The listing builds one solid part. Answer for the finished solid, in the listing's coordinates (mm). Face numbers are marked on the shaded views. A direction names the side the tool comes from. Give positions to 0.01 mm unless a question says otherwise; leave off trailing zeros. Order: outer loops, then holes, each group sorted by start corner. A loop starts at its lowest first (then second) coordinate and runs counter-clockwise, first axis right, second up. Notation, with made-up numbers: (-6.5, 53) - (-2.5, 53) arc R29 cw to (-2.5, 86) - close; hole circle Ø5 at (25, 85.25). An arc over 180 degrees is marked (long way). Use a Markdown table: item, result. Add a question column.
1) The mould has two halves that part along X. Classify the marked faces 5, 6 and 7: released by +X, released by -X, zero draft, split by the parting line, or undercut.
2) Find section D-D, the plane x = 17.5. Determine the outline of the cut face in (y, z), plus the area to 3 significant figures.
3) For the marked faces 1, 2, 3 and 4, determine the directions among +Z, -Z, +X, -X, +Y, -Y from which every point of the face is accessible in a straight line to the end or side of a thin tool.
4) Find section A-A, the plane x = 26.5. Determine the outline of the cut face in (y, z).
5) Find section C-C, the plane z = -4. Determine the outline of the cut face in (x, y).
6) Find section B-B, the plane z = -26.5. Determine the outline of the cut face in (x, y), plus the area to 3 significant figures.
7) Flat-ended cylindrical pins translate along their axes: pin 1 (10 mm diameter, centred on y = 18, z = -20.5, fed in from +X); pin 2 (16.5 mm diameter, centred on y = 11, z = -16.5, fed in from +X); pin 3 (1.5 mm diameter, centred on x = 46, y = 22, fed in from -Z); pin 4 (1.5 mm diameter, centred on x = 6, y = 18.5, fed in from -Z). Find the tip coordinate at first contact, or state that the pin passes through.
8) Straight lines are drawn through the part: line 1 (Z direction, x = 4, y = 4); line 2 (Z direction, x = 67, y = 6); line 3 (Z direction, x = 43.5, y = 19). For each, find the intervals that lie inside material, in ascending order.
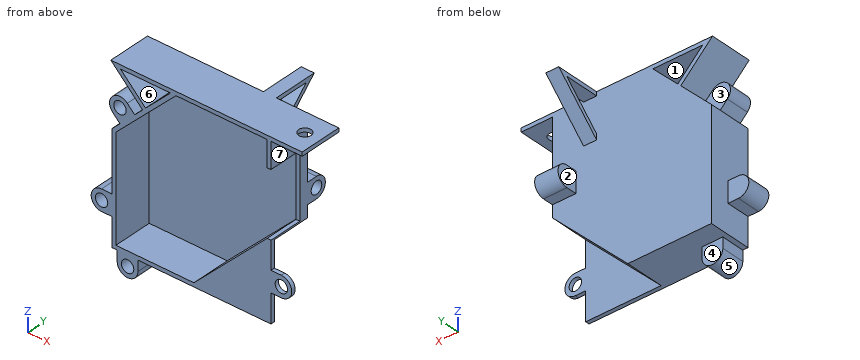
from build123d import *

# Parameters (mm, degrees)
SKETCH1_W            = 38
SKETCH1_H            = 1.5
SKETCH1_W_2          = 1.5
SKETCH1_H_2          = 32
SKETCH1_W_3          = 30
SKETCH1_H_3          = 40
BOSS_EXTRUDE1_DEPTH  = 15
BOSS_EXTRUDE2_DEPTH  = 1.5
SKETCH7_W            = 22
SKETCH7_H            = 12
BOSS_EXTRUDE4_DEPTH  = 10.5
SKETCH9_W            = 12.5
SKETCH9_H            = 8.5
CUT_EXTRUDE10_DEPTH  = 4.5
BOSS_EXTRUDE6_DEPTH  = 1.5
EXTRUDE_THIN1_START  = -20
EXTRUDE_THIN1_DEPTH  = 5
SKETCH16_W           = 10.5
SKETCH16_H           = 12
CUT_EXTRUDE15_DEPTH  = 35.121320344
BOSS_EXTRUDE10_DEPTH = 16
CUT_EXTRUDE16_DEPTH  = 34.560660172
SKETCH21_W           = 1.5
SKETCH21_H           = 25
CUT_EXTRUDE17_DEPTH  = 13
SKETCH25_W           = 1.5
SKETCH25_H           = 16.5
BOSS_EXTRUDE13_DEPTH = 12
BOSS_EXTRUDE14_DEPTH = 9
SKETCH27_R           = 2.38125
CUT_EXTRUDE18_DEPTH  = 6.35
SKETCH29_R           = 2.38125
CUT_EXTRUDE19_DEPTH  = 2.5
BOSS_EXTRUDE15_DEPTH = 9
BOSS_EXTRUDE16_DEPTH = 9
BOSS_EXTRUDE17_DEPTH = 9
BOSS_EXTRUDE18_DEPTH = 1.5
SKETCH34_R           = 2.38125
CUT_EXTRUDE20_DEPTH  = 34.560660172
SKETCH35_R           = 2.38125
CUT_EXTRUDE21_DEPTH  = 6.35


with BuildPart() as part:
    # Sketch1 → Boss-Extrude1 (new body)
    with BuildSketch(Plane(origin=(0, 0, 0), x_dir=(1, 0, 0), z_dir=(0, 1, 0))):
        Polygon((23.112698372, -23.112698372), (0, 0), (-1.060660172, -1.060660172), (10.2760191, -12.397339444), (11.408080409, -13.529400753), (20.991378029, -23.112698372), (22.0520382, -24.173358544), align=None)
        Polygon((23.112698372, -24.612698372), (23.112698372, -23.112698372), (22.0520382, -24.173358544), (22.491378029, -24.612698372), align=None)
        with Locations((42.112698372, -23.862698372)):
            Rectangle(SKETCH1_W, SKETCH1_H)
        with Locations((61.862698372, -23.862698372)):
            Rectangle(SKETCH1_W_2, SKETCH1_H)
        with Locations((61.862698372, -7.112698372)):
            Rectangle(SKETCH1_W_2, SKETCH1_H_2)
        Polygon((62.173358544, 9.9479618), (61.112698372, 8.887301628), (62.612698372, 8.887301628), (62.612698372, 9.508621971), align=None)
        Polygon((31.060660172, 41.060660172), (30, 40), (61.112698372, 8.887301628), (62.173358544, 9.9479618), align=None)
        Polygon((30, 41.5), (30, 40), (31.060660172, 41.060660172), (30.621320344, 41.5), align=None)
        with Locations((15, 40.75)):
            Rectangle(SKETCH1_W_3, SKETCH1_H)
        with Locations((-0.75, 40.75)):
            Rectangle(SKETCH1_W_2, SKETCH1_H)
        with Locations((-0.75, 20)):
            Rectangle(SKETCH1_W_2, SKETCH1_H_3)
        Polygon((-1.060660172, -1.060660172), (0, 0), (-1.5, 0), (-1.5, -0.621320344), align=None)
        Polygon((22.491378029, -24.612698372), (22.0520382, -24.173358544), (20.991378029, -23.112698372), (1.824782789, -23.112698372), (11.408080409, -13.529400753), (10.2760191, -12.397339444), (-1.939339828, -24.612698372), align=None)
    extrude(amount=BOSS_EXTRUDE1_DEPTH)

    # Sketch2 → Boss-Extrude2 (add)
    with BuildSketch(Plane(origin=(0, 15, 0), x_dir=(1, 0, 0), z_dir=(0, 1, 0))):
        Polygon((30.621320344, 41.5), (-1.5, 41.5), (-1.5, -0.621320344), (10.2760191, -12.397339444), (11.408080409, -13.529400753), (20.991378029, -23.112698372), (22.491378029, -24.612698372), (62.612698372, -24.612698372), (62.612698372, 9.508621971), align=None)
        Polygon((0, 40), (30, 40), (61.112698372, 8.887301628), (61.112698372, -23.112698372), (23.112698372, -23.112698372), (0, 0), align=None, mode=Mode.SUBTRACT)
        Polygon((30, 40), (61.112698372, 8.887301628), (61.112698372, -23.112698372), (23.112698372, -23.112698372), (0, 0), (0, 40), align=None)
        Polygon((11.408080409, -13.529400753), (10.2760191, -12.397339444), (-1.939339828, -24.612698372), (19.481361537, -24.612698372), (22.491378029, -24.612698372), (20.991378029, -23.112698372), (1.824782789, -23.112698372), align=None)
    extrude(amount=BOSS_EXTRUDE2_DEPTH)

    # Sketch7 → Boss-Extrude4 (add)
    with BuildSketch(Plane(origin=(62.612698372, 0, 0), x_dir=(0, 0, -1), z_dir=(1, 0, 0))):
        with Locations((-1.491378029, 6)):
            Rectangle(SKETCH7_W, SKETCH7_H)
    extrude(amount=BOSS_EXTRUDE4_DEPTH)

    # Sketch9 → Cut-Extrude10 (cut)
    with BuildSketch(Plane.ZY.offset(-61.112698372)):
        with Locations((1.362698372, 6.25)):
            Rectangle(SKETCH9_W, SKETCH9_H)
    extrude(amount=-CUT_EXTRUDE10_DEPTH, mode=Mode.SUBTRACT)

    # Sketch11 → Boss-Extrude6 (add)
    with BuildSketch(Plane.XZ):
        Polygon((62.612698372, -9.508621971), (30.621320344, -41.5), (62.612698372, -41.5), align=None)
    extrude(amount=-BOSS_EXTRUDE6_DEPTH)

    # Sketch12 → Extrude-Thin1 (add)
    with BuildSketch(Plane(origin=(62.612698372, 0, 0), x_dir=(0, 0, -1), z_dir=(1, 0, 0)).offset(EXTRUDE_THIN1_START)):
        Polygon((-7.5520382, 16.5), (-24.612698372, 33.560660172), (-24.612698372, 16.5), (-23.112698372, 16.5), (-23.112698372, 29.939339828), (-8.612698372, 15.439339828), align=None)
    extrude(amount=EXTRUDE_THIN1_DEPTH)

    # Sketch16 → Cut-Extrude15 (cut, through all)
    with BuildSketch(Plane(origin=(0, 0, -9.508621971), x_dir=(-1, 0, 0), z_dir=(0, 0, -1))):
        with Locations((-67.862698372, 6)):
            Rectangle(SKETCH16_W, SKETCH16_H)
    extrude(amount=-CUT_EXTRUDE15_DEPTH, mode=Mode.SUBTRACT)

    # Sketch19 → Boss-Extrude10 (add)
    with BuildSketch(Plane.XZ):
        Polygon((59.612698372, -10.387301628), (59.612698372, 23.112698372), (58.112698372, 23.112698372), (58.112698372, -11.887301628), align=None)
    extrude(amount=-BOSS_EXTRUDE10_DEPTH)

    # Sketch20 → Cut-Extrude16 (cut, through all)
    with BuildSketch(Plane.XZ):
        Polygon((59.612698372, 23.112698372), (59.612698372, 24.612698372), (62.612698372, 24.612698372), (62.612698372, -41.5), (59.612698372, -41.5), align=None)
    extrude(amount=-CUT_EXTRUDE16_DEPTH, mode=Mode.SUBTRACT)

    # Sketch21 → Cut-Extrude17 (cut)
    with BuildSketch(Plane.XZ):
        with Locations((58.862698372, 0.612698372)):
            Rectangle(SKETCH21_W, SKETCH21_H)
    extrude(amount=-CUT_EXTRUDE17_DEPTH, mode=Mode.SUBTRACT)

    # Sketch25 → Boss-Extrude13 (add)
    with BuildSketch(Plane(origin=(59.612698372, 0, 0), x_dir=(0, 0, -1), z_dir=(1, 0, 0))):
        with Locations((-23.862698372, 8.25)):
            Rectangle(SKETCH25_W, SKETCH25_H)
    extrude(amount=BOSS_EXTRUDE13_DEPTH)

    # Sketch26 → Boss-Extrude14 (add)
    with BuildSketch(Plane(origin=(59.612698372, 0, 0), x_dir=(0, 0, -1), z_dir=(1, 0, 0))):
        with BuildLine():
            Line((-0.112698372, 20.5), (-0.112698372, 16.5))
            Line((-0.112698372, 16.5), (3.887301628, 16.5))
            Line((3.887301628, 16.5), (7.887301628, 16.5))
            Line((7.887301628, 16.5), (7.887301628, 20.5))
            ThreePointArc((7.887301628, 20.5), (3.887301628, 24.5), (-0.112698372, 20.5))
        make_face()
    extrude(amount=-BOSS_EXTRUDE14_DEPTH)

    # Sketch27 → Cut-Extrude18 (cut)
    with BuildSketch(Plane(origin=(59.612698372, 0, 0), x_dir=(0, 0, -1), z_dir=(1, 0, 0))):
        with Locations((3.887301628, 20.5)):
            Circle(SKETCH27_R)
    extrude(amount=-CUT_EXTRUDE18_DEPTH, mode=Mode.SUBTRACT)

    # Sketch29 → Cut-Extrude19 (cut, through all)
    with BuildSketch(Plane(origin=(0, 0, 23.112698372), x_dir=(-1, 0, 0), z_dir=(0, 0, -1))):
        with Locations((-65.612698372, 8.25)):
            Circle(SKETCH29_R)
    extrude(amount=-CUT_EXTRUDE19_DEPTH, mode=Mode.SUBTRACT)

    # Sketch30 → Boss-Extrude15 (add)
    with BuildSketch(Plane.XZ):
        with BuildLine():
            Line((4.5, -41.5), (0.5, -41.5))
            Line((0.5, -41.5), (0.5, -45.5))
            ThreePointArc((0.5, -45.5), (4.5, -49.5), (8.5, -45.5))
            Line((8.5, -45.5), (8.5, -41.5))
            Line((8.5, -41.5), (4.5, -41.5))
        make_face()
    extrude(amount=-BOSS_EXTRUDE15_DEPTH)

    # Sketch31 → Boss-Extrude16 (add)
    with BuildSketch(Plane.XZ):
        with BuildLine():
            Line((-5.5, -30.5), (-1.5, -30.5))
            Line((-1.5, -30.5), (-1.5, -26.5))
            Line((-1.5, -26.5), (-1.5, -22.5))
            Line((-1.5, -22.5), (-5.5, -22.5))
            ThreePointArc((-5.5, -22.5), (-9.5, -26.5), (-5.5, -30.5))
        make_face()
    extrude(amount=-BOSS_EXTRUDE16_DEPTH)

    # Sketch32 → Boss-Extrude17 (add)
    with BuildSketch(Plane.XZ):
        with BuildLine():
            Line((-1.268844699, 6.509329894), (1.559582425, 3.680902769))
            Line((1.559582425, 3.680902769), (4.38800955, 6.509329894))
            Line((4.38800955, 6.509329894), (7.216436675, 9.337757018))
            Line((7.216436675, 9.337757018), (4.38800955, 12.166184143))
            ThreePointArc((4.38800955, 12.166184143), (-1.268844699, 12.166184143), (-1.268844699, 6.509329894))
        make_face()
    extrude(amount=-BOSS_EXTRUDE17_DEPTH)

    # Sketch33 → Boss-Extrude18 (add)
    with BuildSketch(Plane.XZ):
        with BuildLine():
            Line((59.612698372, -26.5), (59.612698372, -30.5))
            Line((59.612698372, -30.5), (63.612698372, -30.5))
            ThreePointArc((63.612698372, -30.5), (67.612698372, -26.5), (63.612698372, -22.5))
            Line((63.612698372, -22.5), (59.612698372, -22.5))
            Line((59.612698372, -22.5), (59.612698372, -26.5))
        make_face()
    extrude(amount=-BOSS_EXTRUDE18_DEPTH)

    # Sketch34 → Cut-Extrude20 (cut, through all)
    with BuildSketch(Plane.XZ):
        with Locations((63.612698372, -26.5)):
            Circle(SKETCH34_R)
    extrude(amount=-CUT_EXTRUDE20_DEPTH, mode=Mode.SUBTRACT)

    # Sketch35 → Cut-Extrude21 (cut)
    with BuildSketch(Plane.XZ):
        with Locations((4.5, -45.5)):
            Circle(SKETCH35_R)
        with Locations((-5.5, -26.5)):
            Circle(SKETCH35_R)
        with Locations((1.559582425, 9.337757018)):
            Circle(SKETCH35_R)
    extrude(amount=-CUT_EXTRUDE21_DEPTH, mode=Mode.SUBTRACT)


solid = part.part
The answers:
| question | item | result |
|---|---|---|
| 1 | face 5 | split by the parting line |
| 1 | face 6 | undercut |
| 1 | face 7 | released by +X |
| 2 | outline | (0, -41.5) - (16.5, -41.5) - (16.5, 19.62) - (0, 19.62) - (0, 17.5) - (15, 17.5) - (15, -40) - (0, -40) - close; (0, 23.11) - (16.5, 23.11) - (16.5, 24.61) - (0, 24.61) - close |
| 2 | area | 171 mm2 |
| 3 | face 1 | +Y, -Y |
| 3 | face 2 | +Z, -Z, -X, +Y |
| 3 | face 3 | -X, +Y |
| 3 | face 4 | -Z, +X, -X, +Y |
| 4 | outline | (0, -41.5) - (16.5, -41.5) - (16.5, 24.61) - (0, 24.61) - (0, 23.11) - (15, 23.11) - (15, -40) - (0, -40) - close |
| 5 | outline | (-1.5, 0) - (0, 0) - (0, 15) - (58.11, 15) - (58.11, 13) - (59.61, 13) - (59.61, 18.12) - (53.26, 18.12) - (53.26, 22.88) - (59.61, 22.88) - (59.61, 24.5) - (50.61, 24.5) - (50.61, 16.5) - (-1.5, 16.5) - close |
| 6 | outline | (-9.5, 0) - (-7.88, 0) - (-7.88, 6.35) - (-3.12, 6.35) - (-3.12, 0) - (0, 0) - (0, 15) - (43.5, 15) - (43.5, 0) - (61.23, 0) - (61.23, 1.5) - (45.62, 1.5) - (45.62, 16.5) - (-1.5, 16.5) - (-1.5, 9) - (-9.5, 9) - close; (65.99, 0) - (67.61, 0) - (67.61, 1.5) - (65.99, 1.5) - close |
| 6 | area | 193 mm2 |
| 7 | pin 1 | x = 56.39 |
| 7 | pin 2 | x = 59.61 |
| 7 | pin 3 | z = 12.3 |
| 7 | pin 4 | through |
| 8 | line 1 | -49.47 to -47.83, -43.17 to -40, 4 to 12.51, 18.67 to 20.94, 23.11 to 24.61 |
| 8 | line 2 | 23.11 to 24.61 |
| 8 | line 3 | 10.05 to 12.17, 23.11 to 24.61 |
